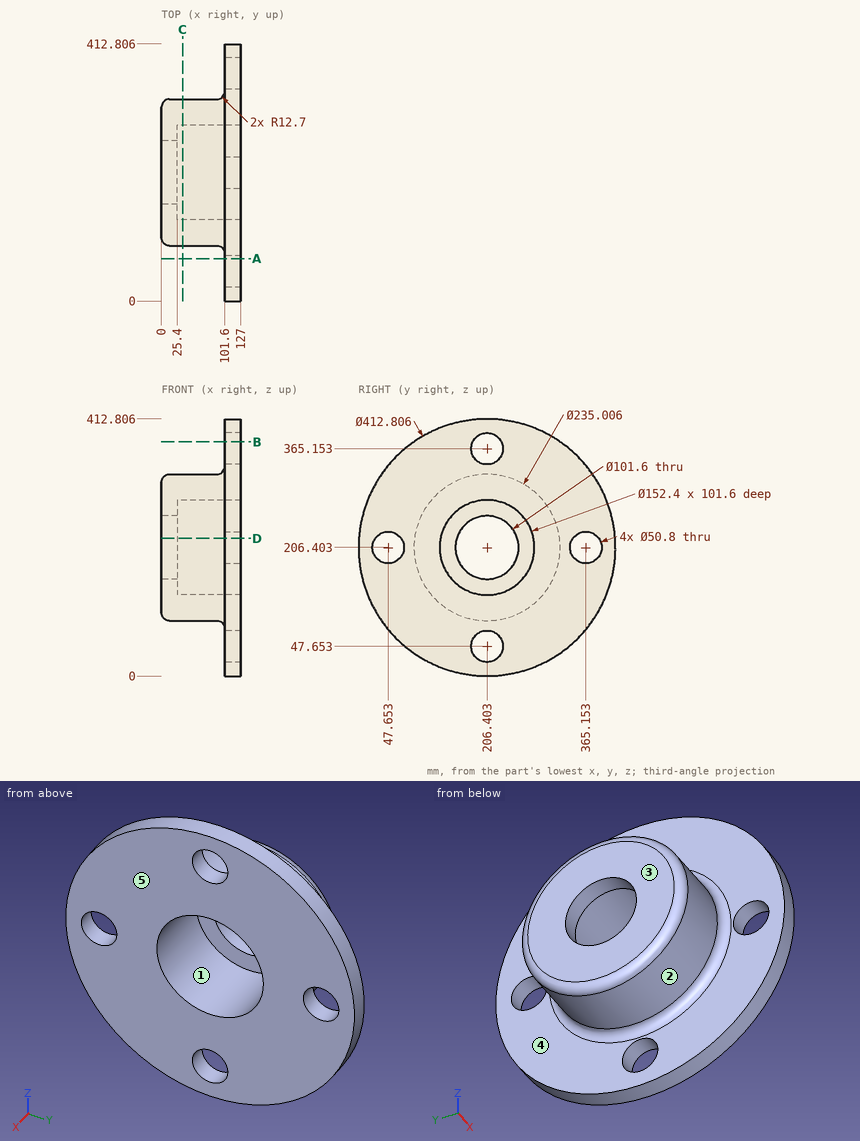
Source: three-view drawing plus pictorial views. Frame: mm from the lowest corner of the part. A direction names the side the tool comes from. Give positions to 0.01 mm unless a question says otherwise; leave off trailing zeros. Loops run counter-clockwise (first coordinate to the right, second up) from the corner with the lowest first, then second, coordinate; pieces in that order, holes last. Notation, with made-up numbers: (26.5, 34.25) -> (42.5, 34.25) arc R21 cw to (42.5, 71.25) -> close; hole circle Ø1 at (19.5, 36.25). An arc over 180 degrees is marked (long way). Put each result on its own line as item: value. Start each with the question number.
1) Reachability of the marked faces 4 and 5 from +Z, -Z, +X, -X, +Y, -Y: full face, straight path, thin tool, end or side. Return the list, or none.
2) Contact query for flat-ended pins moving along their axis: P1, Ø8, axis at y = 230, z = 147.5, coming from the +X side; P2, Ø2, axis at x = 40, z = 277, coming from the -Y side; P3, Ø6, axis at y = 191, z = 292, coming from the -X side; P4, Ø8, axis at x = 62, y = 113.5, coming from the +Z side (1 decimal). Output: stop coordinate, or through.
3) Cut plane A-A (y = 68). Return loops of the section in (x, z).
4) Draft query along Z for the marked faces 1, 2 and 3. Return one class per face: released by +Z, released by -Z, zero draft, split by the parting line, or undercut.
5) Cut plane C-C (x = 34). Return loops of the section in (y, z).
6) Material intervals for probe 1 along Y at (x, z) = (104, 208.5) (1 decimal); probe 2 along X at (y, z) = (149.5, 56.5); probe 3 along Y at (x, z) = (57, 183), sorted ascending.
7) Cut plane D-D (z = 221). State how many separate pieces and enclosed holes the cut face has, then the cut area to 3 significant figures.
8) Cut plane B-B (z = 376). Return loops of the section in (x, y).
Results are:
1. face 4: -X
1. face 5: +Z, -Z, +X, +Y, -Y
2. P1: stops at x = 25.4
2. P2: stops at y = 111.73
2. P3: stops at x = 0
2. P4: stops at z = 283.2
3. outline: (101.6, 53.28) -> (127, 53.28) -> (127, 191.2) -> (101.6, 191.2) -> close; (101.6, 221.61) -> (127, 221.61) -> (127, 359.53) -> (101.6, 359.53) -> close
4. face 1: undercut
4. face 2: split by the parting line
4. face 3: zero draft
5. outline: circle Ø235.01 at (206.4, 206.4); hole circle Ø152.4 at (206.4, 206.4)
6. probe 1: y = 0 to 22.3, 73 to 130.2, 282.6 to 339.8, 390.5 to 412.8
6. probe 2: x = 101.6 to 127
6. probe 3: y = 91.25 to 133.89, 278.92 to 321.55
7. separate pieces: 4
7. enclosed holes: 0
7. area: 14,400 mm2
8. outline: (101.6, 88.76) -> (127, 88.76) -> (127, 183.44) -> (101.6, 183.44) -> close; (101.6, 229.37) -> (127, 229.37) -> (127, 324.04) -> (101.6, 324.04) -> close
